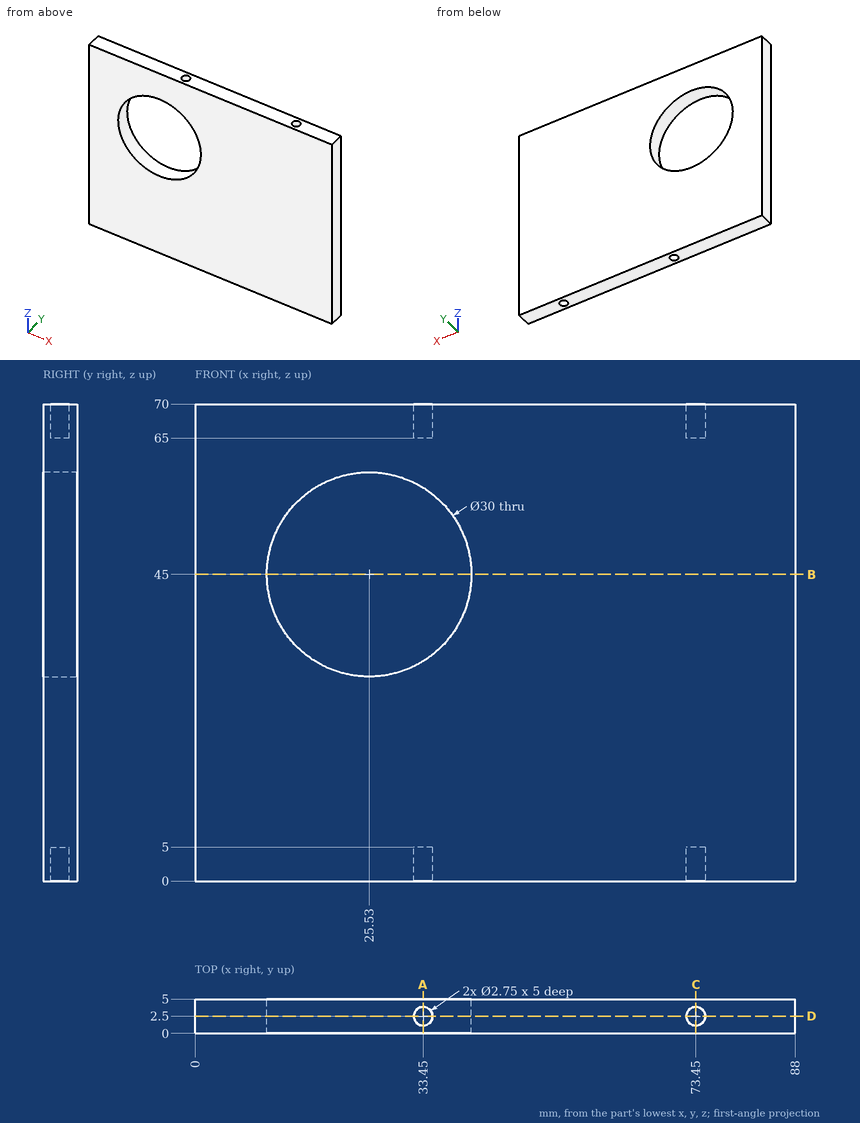
Could you check a few things on this drawing? It's one solid part, dimensions in mm from its lowest x, y, z. Round coordinates to 2 decimals unless told otherwise and drop trailing zeros. Order: outer loops, then holes, each group sorted by start corner. A loop starts at its lowest first (then second) coordinate and runs counter-clockwise, first axis right, second up.
Q1. Imagine slicing it at C-C, the plane x = 73.45. List the corners of the cut face in (y, z) for me (1 decimal).
Geometry says:
outline: (0, 0) - (1.1, 0) - (1.1, 5) - (3.9, 5) - (3.9, 0) - (5, 0) - (5, 70) - (3.9, 70) - (3.9, 65) - (1.1, 65) - (1.1, 70) - (0, 70) - close
Q2. I'm going to push flat-ended pins straight in: P1, Ø0.8, axis at x = 73, y = 2, coming from the +Z side; P2, Ø2, axis at x = 73.45, y = 2.5, coming from the -Z side. Where does each tip first touch, or does it pass through?
Geometry says:
P1: stops at z = 65
P2: stops at z = 5
Q3. Please list where these lines run through material, in increasing order: probe 1 along X at (y, z) = (2.5, 3.8) (1 decimal); probe 2 along Y at (x, z) = (73.45, 2.55) (1 decimal); probe 3 along X at (y, z) = (1.4, 67.5) (1 decimal).
Geometry says:
probe 1: x = 0 to 32.1, 34.8 to 72.1, 74.8 to 88
probe 2: y = 0 to 1.1, 3.9 to 5
probe 3: x = 0 to 32.6, 34.3 to 72.6, 74.3 to 88
Q4. Imagine slicing it at A-A, the plane x = 33.45. List the corners of the cut face in (y, z) for me (1 decimal), then the cut area to 3 significant figures.
Geometry says:
outline: (0, 0) - (1.1, 0) - (1.1, 5) - (3.9, 5) - (3.9, 0) - (5, 0) - (5, 32.3) - (0, 32.3) - close; (0, 57.7) - (5, 57.7) - (5, 70) - (3.9, 70) - (3.9, 65) - (1.1, 65) - (1.1, 70) - (0, 70) - close
area: 195 mm2
Q5. Imagine slicing it at B-B, the plane z = 45. List the corners of the cut face in (x, y) for me.
Geometry says:
outline: (0, 0) - (10.53, 0) - (10.53, 5) - (0, 5) - close; (40.53, 0) - (88, 0) - (88, 5) - (40.53, 5) - close
Q6. Imagine slicing it at D-D, the plane y = 2.5. List the corners of the cut face in (x, z) for me (1 decimal), then the cut area to 3 significant figures.
Geometry says:
outline: (0, 0) - (32.1, 0) - (32.1, 5) - (34.8, 5) - (34.8, 0) - (72.1, 0) - (72.1, 5) - (74.8, 5) - (74.8, 0) - (88, 0) - (88, 70) - (74.8, 70) - (74.8, 65) - (72.1, 65) - (72.1, 70) - (34.8, 70) - (34.8, 65) - (32.1, 65) - (32.1, 70) - (0, 70) - close; hole circle Ø30 at (25.5, 45)
area: 5,400 mm2
